Work out the finished part from the listing and answer in its coordinate system (mm). A direction names the side the tool comes from. Coordinates: 2 decimals unless noted, no trailing zeros. Loops run counter-clockwise (first coordinate to the right, second up) from the corner with the lowest first, then second, coordinate; pieces in that order, holes last. Notation, with made-up numbers: (10.25, 73) -> (28.25, 73) arc R7 ccw to (28.25, 80) -> close; hole circle Ø8 at (-4, 60). An arc over 180 degrees is marked (long way). Use a Markdown table: item, result.
from build123d import *

# Parameters (mm, degrees)
F0_W     = 32.4
F0_H     = 15
F0_R     = 5
F1_DEPTH = 15
F3_D     = 6
F4_D     = 6
F5_DEPTH = 15
F6_DEPTH = 15
F7_D     = 3
F8_D     = 1.5
F8_DEPTH = 3
F8_TIP   = 0.4506454643
F9_D     = 3
F9_DEPTH = 3
F9_TIP   = 0.9012909285
F10_R    = 2
F11_R    = 0.49999


# Not quite as in the source:
# - a fillet or chamfer is up to 0.001 mm smaller than in the source, because OpenCascade refuses the exact size


with BuildPart() as f1:
    # F0 (on Top) → F1 (new body)
    with BuildSketch(Plane.XY):
        Rectangle(F0_W, F0_H)
        Circle(F0_R, mode=Mode.SUBTRACT)
    extrude(amount=F1_DEPTH)

    # F3 (through all)
    with Locations(Plane.XZ.offset(7.5)):
        with Locations((-8.2, 7.5)):
            Hole(F3_D / 2)

    # F4 (through all)
    with Locations(Plane.XZ.offset(7.5)):
        with Locations((8.2, 7.5)):
            Hole(F4_D / 2)

    # F2 (on face) → F5 (cut, through all)
    with BuildSketch(Plane.XZ.offset(7.5)):
        with BuildLine():
            Line((-11.1580398915, 8), (-16.2, 8))
            Line((-16.2, 8), (-16.2, 7.5))
            Line((-16.2, 7.5), (-16.2, 7))
            Line((-16.2, 7), (-11.1580398915, 7))
            ThreePointArc((-11.1580398915, 7), (-11.2, 7.5), (-11.1580398915, 8))
        make_face()
    extrude(amount=-F5_DEPTH, mode=Mode.SUBTRACT)

    # F2 (on face) → F6 (cut, through all)
    with BuildSketch(Plane.XZ.offset(7.5)):
        with BuildLine():
            ThreePointArc((11.1580398915, 8), (11.1894915684, 7.7508787808), (11.2, 7.5))
            ThreePointArc((11.2, 7.5), (11.1894915684, 7.2491212192), (11.1580398915, 7))
            Line((11.1580398915, 7), (16.2, 7))
            Line((16.2, 7), (16.2, 7.5))
            Line((16.2, 7.5), (16.2, 8))
            Line((16.2, 8), (11.1580398915, 8))
        make_face()
    extrude(amount=-F6_DEPTH, mode=Mode.SUBTRACT)

    # F7 (through all)
    with Locations(Plane(origin=(0, 0, 0), x_dir=(1, 0, 0), z_dir=(0, 0, -1))):
        with Locations((-14.2, 0), (14.2, 0)):
            Hole(F7_D / 2)

    # F8
    with Locations(Plane.XZ.offset(7.5)):
        with Locations((0, 7.5)):
            Hole(F8_D / 2, depth=F8_DEPTH)
            with Locations((0, 0, -(F8_DEPTH + F8_TIP / 2))):  # 118° drill point
                Cone(0, F8_D / 2, F8_TIP, mode=Mode.SUBTRACT)

    # F9
    with Locations(Plane.XZ.offset(7.5)):
        with Locations((0, 10.75)):
            Hole(F9_D / 2, depth=F9_DEPTH)
            with Locations((0, 0, -(F9_DEPTH + F9_TIP / 2))):  # 118° drill point
                Cone(0, F9_D / 2, F9_TIP, mode=Mode.SUBTRACT)

    # F10
    f10_edges = [f1.edges().sort_by_distance(p)[0] for p in [
        (16.2, -7.5, 11.5),
        (16.2, -7.5, 3.5),
        (16.2, 7.5, 11.5),
        (16.2, 7.5, 3.5),
        (-16.2, -7.5, 3.5),
        (-16.2, -7.5, 11.5),
        (-16.2, 7.5, 3.5),
        (-16.2, 7.5, 11.5),
    ]]
    fillet(f10_edges, radius=F10_R)

    # F11 (radius 0.5 in the source; OpenCascade refuses exactly that, so slightly less here)
    f11_edges = [f1.edges().sort_by_distance(p)[0] for p in [
        (0, -7.5, 0),
        (0, 7.5, 0),
        (0, -7.5, 15),
        (0, 7.5, 15),
    ]]
    fillet(f11_edges, radius=F11_R)


solid = f1.part
Q1. Section B-B on y = -3 is taken. Determine the outline of the cut face in (x, z), and give its area (3 significant figures).
Solved:
| item | result |
|---|---|
| outline | (-16.2, 0.5) arc R0.5 ccw to (-15.7, 0) -> (-4, 0) -> (-4, 15) -> (-15.7, 15) arc R0.5 ccw to (-16.2, 14.5) -> (-16.2, 8) -> (-11.16, 8) arc R3 cw (long way) to (-11.16, 7) -> (-16.2, 7) -> close; (4, 0) -> (15.7, 0) arc R0.5 ccw to (16.2, 0.5) -> (16.2, 7) -> (11.16, 7) arc R3 cw (long way) to (11.16, 8) -> (16.2, 8) -> (16.2, 14.5) arc R0.5 ccw to (15.7, 15) -> (4, 15) -> close |
| area | 299 mm² |
Q2. Given pin 1 Ø7 at (x, z) = (8.2, 7.5) entering from -Y, flat-ended and moving along its own axis, determine where the tip first touches the part or whether it passes through.
Solved:
| item | result |
|---|---|
| pin 1 | y = -7.5 |
Q3. For faces 4 (the flat face through (0, -7.5, 6)), 5 (the flat face through (-12.5, -0.1, 8)), 6 (the flat face through (12, 0, 8)), determine the directions among +Z, -Z, +X, -X, +Y, -Y from which every point of the face is accessible in a straight line to the end or side of a thin tool.
Solved:
| item | result |
|---|---|
| face 4 | +Z, -Z, +X, -X, -Y |
| face 5 | -X, +Y, -Y |
| face 6 | +X, +Y, -Y |
Q4. Section C-C on z = 1.25 is taken. Determine the outline of the cut face in (x, y).
Solved:
| item | result |
|---|---|
| outline | (-16.2, -5.5) arc R2 ccw to (-14.2, -7.5) -> (14.2, -7.5) arc R2 ccw to (16.2, -5.5) -> (16.2, 5.5) arc R2 ccw to (14.2, 7.5) -> (-14.2, 7.5) arc R2 ccw to (-16.2, 5.5) -> close; hole circle Ø3 at (-14.2, 0); hole circle Ø10 at (0, 0); hole circle Ø3 at (14.2, 0) |
Q5. Determine the mould class of faces 1 (the cylindrical face through (-15.586, 0.575, 11.549)), 2 (the cylindrical face through (-15.63, 6.9, 3.8)), 3 (the flat face through (3, 5, 15)) for opening direction Y: pulls with the +Y half, pulls with the -Y half, needs draft (parallel to the pull), parting line crosses it, or undercut.
Solved:
| item | result |
|---|---|
| face 1 | undercut |
| face 2 | pulls with the +Y half |
| face 3 | needs draft |
Q6. Section D-D on z = 10 is taken. Determine the outline of the cut face in (x, y), and give its area (3 significant figures).
Solved:
| item | result |
|---|---|
| outline | (-16.2, -5.5) arc R2 ccw to (-14.2, -7.5) -> (-9.86, -7.5) -> (-9.86, 7.5) -> (-14.2, 7.5) arc R2 ccw to (-16.2, 5.5) -> close; (-6.54, -7.5) -> (-1.3, -7.5) -> (-1.3, -4.83) arc R5 cw (long way) to (1.3, -4.83) -> (1.3, -7.5) -> (6.54, -7.5) -> (6.54, 7.5) -> (-6.54, 7.5) -> close; (9.86, -7.5) -> (14.2, -7.5) arc R2 ccw to (16.2, -5.5) -> (16.2, 5.5) arc R2 ccw to (14.2, 7.5) -> (9.86, 7.5) -> close; hole circle Ø3 at (-14.2, 0); hole circle Ø3 at (14.2, 0) |
| area | 284 mm² |
Q7. Section A-A on x = 4 is taken. Determine the outline of the cut face in (y, z), and give its area (3 significant figures).
Solved:
| item | result |
|---|---|
| outline | (-7.5, 0.5) arc R0.5 ccw to (-7, 0) -> (-3, 0) -> (-3, 15) -> (-7, 15) arc R0.5 ccw to (-7.5, 14.5) -> close; (3, 0) -> (7, 0) arc R0.5 ccw to (7.5, 0.5) -> (7.5, 14.5) arc R0.5 ccw to (7, 15) -> (3, 15) -> close |
| area | 135 mm² |
Q8. Consider line 1 (Z direction, x = 8.2, y = 0); line 2 (Z direction, x = 13.5, y = -3.5); line 3 (Y direction, x = 14.2, z = 2.75). Determine where each line is inside the solid, lowest interval first. Write a range as [from, to].
Solved:
| item | result |
|---|---|
| line 1 | [0, 4.5], [10.5, 15] |
| line 2 | [0, 7], [8, 15] |
| line 3 | [-7.5, -1.5], [1.5, 7.5] |
